Autodesk Inventor part; units mm, degrees
ref_plane "YZ Plane" through (0, 0, 0) normal (1, 0, 0) x (0, 1, 0)
ref_plane "XZ Plane" through (0, 0, 0) normal (0, 1, 0) x (-1, 0, 0)
ref_plane "XY Plane" through (0, 0, 0) normal (0, 0, 1) x (1, 0, 0)
sketch "Sketch1" plane through (0, 0, 0) normal (0, 0, 1) x (1, 0, 0)
  circle A0 centre (0, 0) radius 28
  circle A1 centre (-20, 0) radius 3.1
  circle A2 centre (-10, -17.3205) radius 3.1
  circle A3 centre (10, -17.3205) radius 3.1
  circle A4 centre (20, 0) radius 3.1
  circle A5 centre (10, 17.3205) radius 3.1
  circle A6 centre (-10, 17.3205) radius 3.1
  dimension "d0" = 56
  dimension "d1" = 6.2
  dimension "d2" = 20
  dimension "d3" = 0
  dimension "d6" = 360
extrude "Extrusion1" add sketch "Sketch1" along normal blind 6
sketch "Sketch2" plane through (0, 0, 0) normal (0, 0, -1) x (-1, 0, 0)
  circle A0 centre (0, 0) radius 15
  dimension "d10" = 30
extrude "Extrusion2" add sketch "Sketch2" along normal blind 20
sketch "Sketch3" plane through (0, 0, 6) normal (0, 0, 1) x (1, 0, 0)
  circle A0 centre (0, 0) radius 28
  circle A1 centre (0, 28) radius 3.05
  circle A2 centre (-24.2487, -14) radius 3.05
  circle A3 centre (24.2487, -14) radius 3.05
  circle A4 centre (0, 8.45) radius 1.55
  line L0 (0, 28) -> (0, 0) construction
  line L1 (0, 0) -> (24.2487, -14) construction
  line L2 (-24.2487, -14) -> (0, 0) construction
  circle A5 centre (7.7509, -4.475) radius 1.05
  circle A6 centre (-7.9674, -4.6) radius 0.8
  circle A7 centre (0, 0) radius 10 construction
  point P0 (25.6276, -11.2795)
  point P1 (22.5821, -16.5544)
  point P2 (-25.6276, -11.2795)
  point P3 (-22.5821, -16.5544)
  point P4 (-3.0455, 27.8339)
  point P5 (3.0455, 27.8339)
  dimension "d13" = 6.1
  dimension "d17" = 360
  dimension "d19" = 3.1
  dimension "d20" = 0
  dimension "d21" = 0
  dimension "d22" = 2.1
  dimension "d23" = 1.6
  dimension "d24" = 20
extrude "Extrusion3" cut sketch "Sketch3" against normal through all contours A1 A0 | A0 A3 | A2 A0 | A4 | A5 | A6 picked at (0.1183, 26.9779) picked at (23.3044, -13.5914) picked at (-23.3241, -13.5486)
chamfer "Chamfer1" distance 2 angle 45 3 edges at (-24.2487, 14, 6) (0, -28, 6) (24.2487, 14, 6)
fillet "Fillet1" radius 1 3 edges at (21.6073, -12.475, 0) (-21.6073, -12.475, 0) (0, 24.95, 0)
properties part number "Schneidtrommel"
The model under review builds one solid part; all positions refer to its coordinate system, in mm. A direction names the side the tool comes from. Round coordinates to 2 decimals unless told otherwise and drop trailing zeros. Loops run counter-clockwise (first coordinate to the right, second up) from the corner with the lowest first, then second, coordinate; pieces in that order, holes last. Notation, with made-up numbers: M 2.25,-34.75 L 35.25,-34.75 A19 ccw 35.25,-28.75 Z; hole C 9.25,88.5 d5. An arc over 180 degrees is marked long. Put each result on its own line as item: value.
Q1. Consider section D-D, the plane z = -5.75. Give the boundary of the cut face in (x, y) (3 decimals), then the cut area to 3 significant figures.
Result set:
outline: C 0,0 d30; hole C -7.967,-4.6 d1.6; hole C 0,8.45 d3.1; hole C 7.751,-4.475 d2.1
area: 694 mm²
Q2. Mouldability with a two-part tool opening along X and no side actions: class faces 3 (the cylindrical face through (-12.46, 19.21, 2.96)), 4 (the flat face through (12, -12, 0)), 5 (the cylindrical face through (24.06, 14.32, 1.97)) as released by +X, released by -X, zero draft, split by the parting line, or undercut.
Result set:
face 3: undercut
face 4: zero draft
face 5: released by +X
Q3. Consider section B-B, the plane z = 1.75. Count the separate pieces of the cut face and the enclosed holes in it, then the cut area to 3 significant figures.
Result set:
separate pieces: 1
enclosed holes: 9
area: 2,230 mm²
Q4. For pin 1 (8 mm diameter, centred on x = -8.5, z = -12, fed in from -Y); pin 2 (2 mm diameter, centred on x = 2.5, z = -15, fed in from -Y); pin 3 (8 mm diameter, centred on x = -10, z = 3, fed in from -Y), all flat-tipped, find the tip position at first contact; note any pin that passes through.
Result set:
pin 1: stops at y = -14.31
pin 2: stops at y = -14.92
pin 3: stops at y = -27.35
Q5. To check wall thickness, follow L1, parallel to X at y = -4.5, z = -14; L2, parallel to Y at x = 10, z = 1.65; L3, parallel to X at y = -18.5, z = 1.75. State the ranges of each line that lie inside material, in increasing order.
Result set:
L1: x = -14.31 to -8.76, -7.17 to 6.7, 8.8 to 14.31
L2: y = -26.15 to -20.42, -14.22 to 14.22, 20.42 to 26.15
L3: x = -21.02 to -12.87, -7.13 to 7.13, 12.87 to 21.02
Q6. Consider section A-A, the plane y = 0. Give the boundary of the cut face in (x, z), then the cut area to 3 significant figures.
Result set:
outline: M -28,0 L -23.1,0 L -23.1,6 L -26,6 L -28,4 Z; M -16.9,0 L -15,0 L -15,-20 L 15,-20 L 15,0 L 16.9,0 L 16.9,6 L -16.9,6 Z; M 23.1,0 L 28,0 L 28,4 L 26,6 L 23.1,6 Z
area: 858 mm²
Q7. Machinability: for faces 1 (the cylindrical face through (-12.46, -15.434, 2.958)), 2 (the cylindrical face through (14.985, -0.66, -9.86)), which of the approach directions +Z, -Z, +X, -X, +Y, -Y give a long, thin tool a straight path to every point of the face, cutting with its end or side? Answer none if there is none.
Result set:
face 1: +Z, -Z
face 2: -Z
